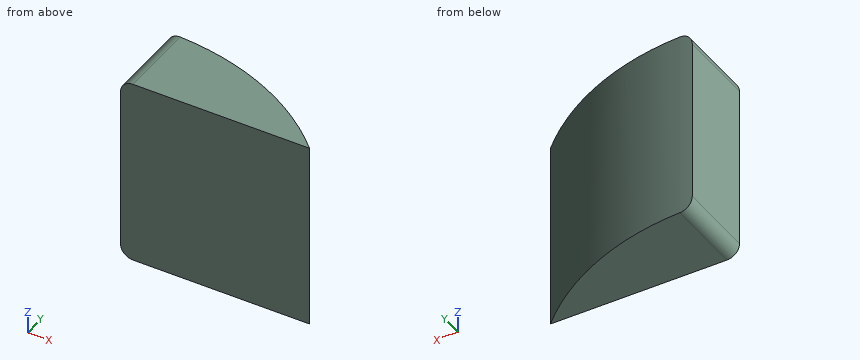
Autodesk Inventor part; units mm, degrees
ref_plane "YZ Plane" through (0, 0, 0) normal (1, 0, 0) x (0, 1, 0)
ref_plane "XZ Plane" through (0, 0, 0) normal (0, 1, 0) x (-1, 0, 0)
ref_plane "XY Plane" through (0, 0, 0) normal (0, 0, 1) x (1, 0, 0)
sketch "Sketch1" plane through (0, 0, 0) normal (0, 0, 1) x (1, 0, 0)
  line L0 (-15, -6.25) -> (15, -6.25)
  line L1 (15, -6.25) -> (15, 6.25)
  line L2 (15, 6.25) -> (-15, 6.25)
  line L3 (-15, 6.25) -> (-15, -6.25)
  line L4 (-15, -6.25) -> (15, 6.25) construction
  line L5 (15, -6.25) -> (-15, 6.25) construction
  arc A0 (15, -6.25) -> (-15, 6.25) centre (-15, -36) ccw
  point P0 (0, 0)
  dimension "d0" = 30
  dimension "d1" = 12.5
extrude "Extrusion1" add sketch "Sketch1" along normal blind 30 contours L3 A0 L0
fillet "Fillet1" radius 2 2 edges at (-15, 0, 30) (-15, 0, 0)
properties part number "linear_stop_brackets"
The model under review builds one solid part; all positions refer to its coordinate system, in mm. Round coordinates to 2 decimals unless told otherwise and drop trailing zeros. Loops run counter-clockwise (first coordinate to the right, second up) from the corner with the lowest first, then second, coordinate; pieces in that order, holes last. Notation, with made-up numbers: M -16.5,79 L 21.5,79 A25 ccw 21.5,105 Z; hole C 53,-26.75 d9. An arc over 180 degrees is marked long. Put each result on its own line as item: value.
Q1. For pin 1 (5 mm diameter, centred on x = -8.5, y = -1, fed in from -Z); pin 2 (5 mm diameter, centred on x = 1, z = 4.5, fed in from +Y); pin 3 (5 mm diameter, centred on y = 5, z = 4, fed in from +X), all flat-tipped, find the tip position at first contact; note any pin that passes through.
Result set:
pin 1: stops at z = 0
pin 2: stops at y = 4.04
pin 3: stops at x = 2.4
Q2. Consider section D-D, the plane y = -5. Give the boundary of the cut face in (x, z).
Result set:
outline: M -15,2 A2 ccw -13,0 L 13.71,0 L 13.71,30 L -13,30 A2 ccw -15,28 Z
Q3. Consider section B-B, the plane z = 15. Give the boundary of the cut face in (x, y).
Result set:
outline: M -15,-6.25 L 15,-6.25 A42.25 ccw -15,6.25 Z
Q4. Consider section C-C, the plane x = -9. Give the boundary of the cut face in (y, z).
Result set:
outline: M -6.25,0 L 5.82,0 L 5.82,30 L -6.25,30 Z
Q5. Consider section A-A, the plane y = 4. Give the boundary of the cut face in (x, z).
Result set:
outline: M -15,2 A2 ccw -13,0 L -1.4,0 L -1.4,30 L -13,30 A2 ccw -15,28 Z
Q6. To check wall thickness, follow L1, parallel to X at y = 3, z = 6.5; L2, parallel to Y at x = -4.5, z = 3; L3, parallel to Y at x = 2, z = 27.5. State the ranges of each line that lie inside material, in increasing order.
Result set:
L1: x = -15 to 1.25
L2: y = -6.25 to 4.92
L3: y = -6.25 to 2.68
